Here's how the part is built. I have some questions about the finished solid (model axes, mm). A direction names the side the tool comes from. Round coordinates to 2 decimals unless told otherwise and drop trailing zeros. Order: outer loops, then holes, each group sorted by start corner. A loop starts at its lowest first (then second) coordinate and runs counter-clockwise, first axis right, second up.
Autodesk Inventor part; units mm, degrees
ref_plane "YZ Plane" through (0, 0, 0) normal (1, 0, 0) x (0, 1, 0)
ref_plane "XZ Plane" through (0, 0, 0) normal (0, 1, 0) x (-1, 0, 0)
ref_plane "XY Plane" through (0, 0, 0) normal (0, 0, 1) x (1, 0, 0)
sketch "Sketch1" plane through (0, 0, 0) normal (0, 1, 0) x (-1, 0, 0)
  circle A0 centre (0, 0) radius 12.5
  dimension "d0" = 25
extrude "Extrusion1" add sketch "Sketch1" along normal blind 3
sketch "Sketch2" plane through (0, 3, 0) normal (0, 1, 0) x (1, 0, 0)
  circle A0 centre (0, 0) radius 16
  dimension "d3" = 32
extrude "Extrusion2" add sketch "Sketch2" along normal blind 2
sketch "Sketch3" plane through (0, 0, 0) normal (0, -1, 0) x (1, 0, 0)
  circle A0 centre (0, 0) radius 16
  dimension "d6" = 32
extrude "Extrusion3" add sketch "Sketch3" along normal blind 2
sketch "Sketch4" plane through (0, -2, 0) normal (0, -1, 0) x (1, 0, 0)
  circle A0 centre (0, 0) radius 2.5
  dimension "d9" = 5
extrude "Extrusion4" cut sketch "Sketch4" against normal through all
properties part number "reverse gear piston"
1. If we section it at B-B, the plane z = 0: Write out the boundary of the cut face in (x, y).
Evaluation:
outline: (-16, -2) - (-2.5, -2) - (-2.5, 5) - (-16, 5) - (-16, 3) - (-12.5, 3) - (-12.5, 0) - (-16, 0) - close; (2.5, -2) - (16, -2) - (16, 0) - (12.5, 0) - (12.5, 3) - (16, 3) - (16, 5) - (2.5, 5) - close
2. I need wall thicknesses on probe 1 along Y at (x, z) = (-8.5, -13); probe 2 along Z at (x, y) = (0, 2.25); probe 3 along Z at (x, y) = (0, 3.5). Which ranges of each line are inside material? Lowest first, please.
Evaluation:
probe 1: y = -2 to 0, 3 to 5
probe 2: z = -12.5 to -2.5, 2.5 to 12.5
probe 3: z = -16 to -2.5, 2.5 to 16
3. If we mould it in two halves opening along Z, with no side actions, what happens to faces 1 (the cylindrical face through (-11.923, 1.479, -3.755)), 2 (the cylindrical face through (-0.54, 1.45, -2.44)), 3 (the flat face through (-10, 0, -8))? For each: released by +Z, released by -Z, zero draft, split by the parting line, or undercut.
Evaluation:
face 1: split by the parting line
face 2: undercut
face 3: zero draft
4. If we section it at A-A, the plane x = 0: Write out the boundary of the cut face in (y, z), and give its area (3 significant figures).
Evaluation:
outline: (-2, -16) - (0, -16) - (0, -12.5) - (3, -12.5) - (3, -16) - (5, -16) - (5, -2.5) - (-2, -2.5) - close; (-2, 2.5) - (5, 2.5) - (5, 16) - (3, 16) - (3, 12.5) - (0, 12.5) - (0, 16) - (-2, 16) - close
area: 168 mm2
5. If we section it at C-C, the plane y = -0.5: Write out the boundary of the cut face in (x, z), and give its area (3 significant figures).
Evaluation:
outline: circle Ø32 at (0, 0); hole circle Ø5 at (0, 0)
area: 785 mm2
6. I'm going to push flat-ended pins straight in: P1, Ø3, axis at y = 2, z = 9.5, coming from the +X side; P2, Ø1.5, axis at y = 0, z = -8, coming from the +X side; P3, Ø3, axis at y = -0.5, z = 9.5, coming from the -X side. Where does each tip first touch, or does it pass through?
Evaluation:
P1: stops at x = 13.63
P2: stops at x = 14.26
P3: stops at x = -13.86
7. On a 3-axis mill with a long thin cutter (end or side, diameter ignored), from which of +Z, -Z, +X, -X, +Y, -Y can I reach the whole of each face in a straight line? I mean faces 4 (the flat face through (-10, 3, 8)), 5 (the cylindrical face through (-3.47, 3.99, -15.62)). Say none if no direction works.
Evaluation:
face 4: none
face 5: +Y, -Y
8. If we section it at D-D, the plane z = 4: Write out the boundary of the cut face in (x, y).
Evaluation:
outline: (-15.49, -2) - (15.49, -2) - (15.49, 0) - (11.84, 0) - (11.84, 3) - (15.49, 3) - (15.49, 5) - (-15.49, 5) - (-15.49, 3) - (-11.84, 3) - (-11.84, 0) - (-15.49, 0) - close
